The listing builds one solid part. Answer for the finished solid, in the listing's coordinates (mm). Round coordinates to 2 decimals unless told otherwise and drop trailing zeros. Loops run counter-clockwise (first coordinate to the right, second up) from the corner with the lowest first, then second, coordinate; pieces in that order, holes last. Notation, with made-up numbers: (-40, 36.5) -> (-22, 36.5) arc R15 ccw to (-22, 60.5) -> close; hole circle Ø3 at (-9, 36.25). An arc over 180 degrees is marked (long way). Write each question's results on one line, items separated by ' | '. Start each with the question number.
(1) A flat-ended cylindrical pin translates along its axis: pin 1 (6 mm diameter, centred on x = -20, z = 20, fed in from -Y). Find the tip coordinate at first contact, or state that the pin passes through.
(2) The part is cut by section B-B (z = -10). Determine the outline of the cut face in (x, y).
(3) Straight lines are drawn through the part: probe 1 along X at (y, z) = (2.3, 20); probe 2 along X at (y, z) = (1.45, 0); probe 3 along X at (y, z) = (0.95, 10). For each, find the intervals that lie inside material, in ascending order.
(4) The part is cut by section D-D (x = -9). Determine the outline of the cut face in (y, z).
(5) The part is cut by section A-A (x = 20). Count the separate pieces of the cut face and the enclosed holes in it, plus the area to 3 significant figures.
(6) The part is cut by section C-C (z = 0). Determine the outline of the cut face in (x, y).
```python
from build123d import *

# Parameters (mm, degrees)
SKETCH1_W           = 65.5
SKETCH1_H           = 65.5
SKETCH1_R           = 3.6
SKETCH1_R_2         = 2.55
BOSS_EXTRUDE1_DEPTH = 3
FILLET2_R           = 3


with BuildPart() as part:
    # Sketch1 → Boss-Extrude1 (new body)
    with BuildSketch(Plane(origin=(0, 0, 0), x_dir=(1, 0, 0), z_dir=(0, 1, 0))):
        Rectangle(SKETCH1_W, SKETCH1_H)
        with BuildLine():
            Line((-16.9, -29.191507266), (-16.9, -29.2))
            Line((-16.9, -29.2), (-23.4, -29.2))
            ThreePointArc((-23.4, -29.2), (-24.9, -27.7), (-23.4, -26.2))
            Line((-23.4, -26.2), (-16.9, -26.2))
            Line((-16.9, -26.2), (-16.9, -26.208492734))
            ThreePointArc((-16.9, -26.208492734), (-15.845345098, -26.645345098), (-15.408492734, -27.7))
            ThreePointArc((-15.408492734, -27.7), (-15.845345098, -28.754654902), (-16.9, -29.191507266))
        make_face(mode=Mode.SUBTRACT)
        with Locations((-20, -20)):
            Circle(SKETCH1_R, mode=Mode.SUBTRACT)
        with BuildLine():
            Line((-3.25, -26.2), (3.25, -26.2))
            Line((3.25, -26.2), (3.25, -26.208492734))
            ThreePointArc((3.25, -26.208492734), (4.304654902, -26.645345098), (4.741507266, -27.7))
            ThreePointArc((4.741507266, -27.7), (4.304654902, -28.754654902), (3.25, -29.191507266))
            Line((3.25, -29.191507266), (3.25, -29.2))
            Line((3.25, -29.2), (-3.25, -29.2))
            ThreePointArc((-3.25, -29.2), (-4.75, -27.7), (-3.25, -26.2))
        make_face(mode=Mode.SUBTRACT)
        with BuildLine():
            Line((-10.32, -17.5), (10.32, -17.5))
            ThreePointArc((10.32, -17.5), (12.087766953, -18.232233047), (12.82, -20))
            ThreePointArc((12.82, -20), (12.087766953, -21.767766953), (10.32, -22.5))
            Line((10.32, -22.5), (-10.32, -22.5))
            ThreePointArc((-10.32, -22.5), (-12.82, -20), (-10.32, -17.5))
        make_face(mode=Mode.SUBTRACT)
        with Locations((-20, -10)):
            Circle(SKETCH1_R_2, mode=Mode.SUBTRACT)
        with Locations((0, -10)):
            Circle(SKETCH1_R_2, mode=Mode.SUBTRACT)
        with BuildLine():
            Line((23.4, -29.191507266), (23.4, -29.2))
            Line((23.4, -29.2), (16.9, -29.2))
            ThreePointArc((16.9, -29.2), (15.4, -27.7), (16.9, -26.2))
            Line((16.9, -26.2), (23.4, -26.2))
            Line((23.4, -26.2), (23.4, -26.208492734))
            ThreePointArc((23.4, -26.208492734), (24.454654902, -26.645345098), (24.891507266, -27.7))
            ThreePointArc((24.891507266, -27.7), (24.454654902, -28.754654902), (23.4, -29.191507266))
        make_face(mode=Mode.SUBTRACT)
        with Locations((20, -20)):
            Circle(SKETCH1_R_2, mode=Mode.SUBTRACT)
        Circle(SKETCH1_R_2, mode=Mode.SUBTRACT)
        with Locations((20, -10)):
            Circle(SKETCH1_R_2, mode=Mode.SUBTRACT)
        with Locations((-20, 0)):
            Circle(SKETCH1_R_2, mode=Mode.SUBTRACT)
        with Locations((-20, 10)):
            Circle(SKETCH1_R_2, mode=Mode.SUBTRACT)
        with Locations((-10, 0)):
            Circle(SKETCH1_R_2, mode=Mode.SUBTRACT)
        with Locations((-20, 20)):
            Circle(SKETCH1_R, mode=Mode.SUBTRACT)
        with BuildLine():
            Line((-23.4, 29.2), (-16.9, 29.2))
            Line((-16.9, 29.2), (-16.9, 29.191507266))
            ThreePointArc((-16.9, 29.191507266), (-15.845345098, 28.754654902), (-15.408492734, 27.7))
            ThreePointArc((-15.408492734, 27.7), (-15.845345098, 26.645345098), (-16.9, 26.208492734))
            Line((-16.9, 26.208492734), (-16.9, 26.2))
            Line((-16.9, 26.2), (-23.4, 26.2))
            ThreePointArc((-23.4, 26.2), (-24.9, 27.7), (-23.4, 29.2))
        make_face(mode=Mode.SUBTRACT)
        with BuildLine():
            Line((-10.32, 22.5), (10.32, 22.5))
            ThreePointArc((10.32, 22.5), (12.087766953, 21.767766953), (12.82, 20))
            ThreePointArc((12.82, 20), (12.087766953, 18.232233047), (10.32, 17.5))
            Line((10.32, 17.5), (-10.32, 17.5))
            ThreePointArc((-10.32, 17.5), (-12.82, 20), (-10.32, 22.5))
        make_face(mode=Mode.SUBTRACT)
        with BuildLine():
            Line((-3.25, 29.2), (3.25, 29.2))
            Line((3.25, 29.2), (3.25, 29.191507266))
            ThreePointArc((3.25, 29.191507266), (4.304654902, 28.754654902), (4.741507266, 27.7))
            ThreePointArc((4.741507266, 27.7), (4.304654902, 26.645345098), (3.25, 26.208492734))
            Line((3.25, 26.208492734), (3.25, 26.2))
            Line((3.25, 26.2), (-3.25, 26.2))
            ThreePointArc((-3.25, 26.2), (-4.75, 27.7), (-3.25, 29.2))
        make_face(mode=Mode.SUBTRACT)
        with Locations((10, 0)):
            Circle(SKETCH1_R_2, mode=Mode.SUBTRACT)
        with Locations((0, 10)):
            Circle(SKETCH1_R_2, mode=Mode.SUBTRACT)
        with Locations((20, 0)):
            Circle(SKETCH1_R_2, mode=Mode.SUBTRACT)
        with Locations((20, 10)):
            Circle(SKETCH1_R_2, mode=Mode.SUBTRACT)
        with Locations((20, 20)):
            Circle(SKETCH1_R_2, mode=Mode.SUBTRACT)
        with BuildLine():
            Line((16.9, 29.2), (23.4, 29.2))
            Line((23.4, 29.2), (23.4, 29.191507266))
            ThreePointArc((23.4, 29.191507266), (24.454654902, 28.754654902), (24.891507266, 27.7))
            ThreePointArc((24.891507266, 27.7), (24.454654902, 26.645345098), (23.4, 26.208492734))
            Line((23.4, 26.208492734), (23.4, 26.2))
            Line((23.4, 26.2), (16.9, 26.2))
            ThreePointArc((16.9, 26.2), (15.4, 27.7), (16.9, 29.2))
        make_face(mode=Mode.SUBTRACT)
    extrude(amount=BOSS_EXTRUDE1_DEPTH)

    # Fillet2
    fillet2_edges = [part.edges().sort_by_distance(p)[0] for p in [
        (-32.75, 1.5, -32.75),
        (32.75, 1.5, -32.75),
        (32.75, 1.5, 32.75),
        (-32.75, 1.5, 32.75),
    ]]
    fillet(fillet2_edges, radius=FILLET2_R)


solid = part.part
```
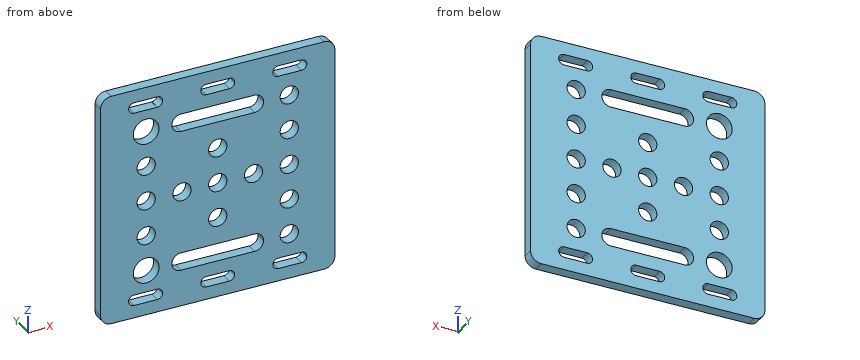
Checked values:
1) pin 1: passes through
2) outline: (-32.75, 0) -> (-22.55, 0) -> (-22.55, 3) -> (-32.75, 3) -> close; (-17.45, 0) -> (-2.55, 0) -> (-2.55, 3) -> (-17.45, 3) -> close; (2.55, 0) -> (17.45, 0) -> (17.45, 3) -> (2.55, 3) -> close; (22.55, 0) -> (32.75, 0) -> (32.75, 3) -> (22.55, 3) -> close
3) probe 1: x = -32.75 to -23.6, -16.4 to -12.82, 12.82 to 17.45, 22.55 to 32.75 | probe 2: x = -32.75 to -22.55, -17.45 to -12.55, -7.45 to -2.55, 2.55 to 7.45, 12.55 to 17.45, 22.55 to 32.75 | probe 3: x = -32.75 to -22.55, -17.45 to -2.55, 2.55 to 17.45, 22.55 to 32.75
4) outline: (0, -32.75) -> (3, -32.75) -> (3, -22.5) -> (0, -22.5) -> close; (0, -17.5) -> (3, -17.5) -> (3, -2.35) -> (0, -2.35) -> close; (0, 2.35) -> (3, 2.35) -> (3, 17.5) -> (0, 17.5) -> close; (0, 22.5) -> (3, 22.5) -> (3, 32.75) -> (0, 32.75) -> close
5) separate pieces: 8 | enclosed holes: 0 | area: 102 mm2
6) outline: (-32.75, 0) -> (-22.55, 0) -> (-22.55, 3) -> (-32.75, 3) -> close; (-17.45, 0) -> (-12.55, 0) -> (-12.55, 3) -> (-17.45, 3) -> close; (-7.45, 0) -> (-2.55, 0) -> (-2.55, 3) -> (-7.45, 3) -> close; (2.55, 0) -> (7.45, 0) -> (7.45, 3) -> (2.55, 3) -> close; (12.55, 0) -> (17.45, 0) -> (17.45, 3) -> (12.55, 3) -> close; (22.55, 0) -> (32.75, 0) -> (32.75, 3) -> (22.55, 3) -> close
